Read the model definition and answer for the solid it produces. Units are mm, in the model's axes. Give positions to 0.01 mm unless a question says otherwise; leave off trailing zeros. Loops run counter-clockwise (first coordinate to the right, second up) from the corner with the lowest first, then second, coordinate; pieces in that order, holes last. Notation, with made-up numbers: (47, -32) - (69, -32) arc R15 ccw to (69, -16) - close; hole circle Ø11 at (48.25, 85.5). An arc over 180 degrees is marked (long way). Put each result on its own line as item: value. Start each with the question number.
1. A cutting plane is placed at A-A, the plane x = 197. Determine the outline of the cut face in (y, z), plus the area to 3 significant figures.
2. For a pull along Y with two mould halves and no side action, classify faces 1 (the cylindrical face through (175.95, 99.06, 2.35)), 2 (the flat face through (187.261, 108.977, 2.348)), 3 (the cylindrical face through (194.393, 85.716, 2.348)) as released by +Y, released by -Y, zero draft, split by the parting line, or undercut.
3. Consider L1, parallel to X at y = 96.5, z = 1; L2, parallel to Y at x = 200.5, z = 3.9; L3, parallel to Y at x = 198.5, z = 4.5. Determine where each line is inside the solid, lowest interval first. Write a range as from..to.
4. A cutting plane is placed at D-D, the plane y = 109. Determine the outline of the cut face in (x, z), plus the area to 3 significant figures.
5. A cutting plane is placed at C-C, the plane x = 182. Determine the outline of the cut face in (y, z).
6. A cutting plane is placed at B-B, the plane y = 95.5. Determine the outline of the cut face in (x, z).
7. Given pin 1 Ø1.5 at (x, z) = (192, 1.5) entering from +Y; pin 2 Ø2 at (x, z) = (190.5, 1.5) entering from -Y, each flat-ended and moving along its own axis, determine where each tip first touches the part or whether it passes through.
```python
from build123d import *

# Parameters (mm, degrees)
SKETCH1_R           = 6.00075
SKETCH1_R_2         = 1.6
SKETCH1_R_3         = 6.6
BOSS_EXTRUDE1_DEPTH = 4.7625


with BuildPart() as part:
    # Sketch1 → Boss-Extrude1 (new body)
    with BuildSketch(Plane.XY):
        with BuildLine():
            Line((179.148086511, 103.607144631), (195.603327806, 114.500302414))
            ThreePointArc((195.603327806, 114.500302414), (198.919543637, 115.552562907), (202.292483355, 114.699440851))
            Line((202.292483355, 114.699440851), (211.27381454, 109.494480567))
            ThreePointArc((211.27381454, 109.494480567), (219.765287832, 91.502488859), (205.940797496, 77.195135812))
            Line((205.940797496, 77.195135812), (205.873802068, 77.181697321))
            ThreePointArc((205.873802068, 77.181697321), (189.799923624, 79.228940232), (178.234639917, 90.578168601))
            ThreePointArc((178.234639917, 90.578168601), (177.435417915, 92.133945768), (176.622616151, 93.682671597))
            ThreePointArc((176.622616151, 93.682671597), (175.969639562, 99.132397301), (179.148086511, 103.607144631))
        make_face()
        with Locations((184.517388009, 97.618855822)):
            Circle(SKETCH1_R, mode=Mode.SUBTRACT)
        with Locations((199.571302743, 106.841754978)):
            Circle(SKETCH1_R, mode=Mode.SUBTRACT)
        with Locations((212.083037321, 102.378153756)):
            Circle(SKETCH1_R_2, mode=Mode.SUBTRACT)
        with Locations((210.523861298, 84.769378384)):
            Circle(SKETCH1_R_2, mode=Mode.SUBTRACT)
        with Locations((192.915085926, 86.328554406)):
            Circle(SKETCH1_R_2, mode=Mode.SUBTRACT)
        with Locations((202.499061623, 94.353354081)):
            Circle(SKETCH1_R_3, mode=Mode.SUBTRACT)
    extrude(amount=BOSS_EXTRUDE1_DEPTH)


solid = part.part
```
Return value:
1. outline: (76.98, 0) - (90.7, 0) - (90.7, 4.76) - (76.98, 4.76) - close; (98, 0) - (101.42, 0) - (101.42, 4.76) - (98, 4.76) - close; (112.26, 0) - (115.2, 0) - (115.2, 4.76) - (112.26, 4.76) - close
1. area: 95.6 mm2
2. face 1: split by the parting line
2. face 2: released by +Y
2. face 3: undercut
3. L1: x = 175.77..178.62, 190.41..196.26, 208.74..219.87
3. L2: y = 76.69..88.06, 100.64..100.91, 112.77..115.4
3. L3: y = 76.8..89.1, 99.6..100.94, 112.75..115.53
4. outline: (187.29, 0) - (193.97, 0) - (193.97, 4.76) - (187.29, 4.76) - close; (205.17, 0) - (212.08, 0) - (212.08, 4.76) - (205.17, 4.76) - close
4. area: 64.7 mm2
5. outline: (85.09, 0) - (92.17, 0) - (92.17, 4.76) - (85.09, 4.76) - close; (103.07, 0) - (105.5, 0) - (105.5, 4.76) - (103.07, 4.76) - close
6. outline: (175.94, 0) - (178.9, 0) - (178.9, 4.76) - (175.94, 4.76) - close; (190.13, 0) - (196, 0) - (196, 4.76) - (190.13, 4.76) - close; (209, 0) - (219.96, 0) - (219.96, 4.76) - (209, 4.76) - close
7. pin 1: stops at y = 112.61
7. pin 2: stops at y = 78.48
